Autodesk Inventor part; units mm, degrees
ref_plane "YZ Plane" through (0, 0, 0) normal (1, 0, 0) x (0, 1, 0)
ref_plane "XZ Plane" through (0, 0, 0) normal (0, 1, 0) x (-1, 0, 0)
ref_plane "XY Plane" through (0, 0, 0) normal (0, 0, 1) x (1, 0, 0)
sketch "Sketch1" plane through (0, 0, 0) normal (1, 0, 0) x (0, 1, 0)
  circle A0 centre (0, 0) radius 22.5
  circle A1 centre (0, 0) radius 8.375
  line L0 (8.375, 0) -> (22.5, 0) construction
  line L1 (22.1638, 3.875) -> (7.4246, 3.875) construction
  line L2 (7.4246, -3.875) -> (22.1638, -3.875) construction
  circle A2 centre (-14, 0) radius 3.0375
  circle A3 centre (-4.3262, -13.3148) radius 3.0375
  circle A4 centre (11.3262, -8.229) radius 3.0375
  circle A5 centre (11.3262, 8.229) radius 3.0375
  circle A6 centre (-4.3262, 13.3148) radius 3.0375
  dimension "d0" = 45
  dimension "d1" = 16.75
  dimension "d2" = 7.75
  dimension "d3" = 3.875
  dimension "d4" = 0
  dimension "d5" = 6.075
  dimension "d32" = 14
  dimension "d35" = 360
extrude "Extrusion1" add sketch "Sketch1" along normal blind 2
sketch "Sketch2" plane through (0, 0, 0) normal (-1, 0, 0) x (0, 0, 1)
  circle A0 centre (0, 0) radius 8.375
  circle A1 centre (0, 0) radius 22.5
extrude "Extrusion2" add sketch "Sketch2" along normal blind 0.25
sketch "Sketch3" plane through (2, 0, 0) normal (1, 0, 0) x (0, 0, -1)
  line L0 (-3.1, 26.8099) -> (3.1, 26.8099)
  line L1 (3.1, 26.8099) -> (3.1, 14.5)
  line L2 (3.1, 14.5) -> (-3.1, 14.5)
  line L3 (-3.1, 14.5) -> (-3.1, 26.8099)
  circle A0 centre (0, 0) radius 22.5 construction
  line L4 (-2.05, 26.8099) -> (2.05, 26.8099)
  line L5 (2.05, 26.8099) -> (2.05, 14.5)
  line L6 (2.05, 14.5) -> (-2.05, 14.5)
  line L7 (-2.05, 14.5) -> (-2.05, 26.8099)
  line L8 (-26.4557, 5.3365) -> (-24.5398, 11.233)
  line L9 (-24.5398, 11.233) -> (-12.8324, 7.429)
  line L10 (-12.8324, 7.429) -> (-14.7483, 1.5325)
  line L11 (-14.7483, 1.5325) -> (-26.4557, 5.3365)
  line L12 (-26.1313, 6.3351) -> (-24.8643, 10.2344)
  line L13 (-24.8643, 10.2344) -> (-13.1568, 6.4304)
  line L14 (-13.1568, 6.4304) -> (-14.4238, 2.5311)
  line L15 (-14.4238, 2.5311) -> (-26.1313, 6.3351)
  line L16 (-13.2505, -23.5118) -> (-18.2664, -19.8676)
  line L17 (-18.2664, -19.8676) -> (-11.0308, -9.9086)
  line L18 (-11.0308, -9.9086) -> (-6.0149, -13.5529)
  line L19 (-6.0149, -13.5529) -> (-13.2505, -23.5118)
  line L20 (-14.1, -22.8947) -> (-17.417, -20.4847)
  line L21 (-17.417, -20.4847) -> (-10.1814, -10.5258)
  line L22 (-10.1814, -10.5258) -> (-6.8644, -12.9357)
  line L23 (-6.8644, -12.9357) -> (-14.1, -22.8947)
  line L24 (18.2664, -19.8676) -> (13.2505, -23.5118)
  line L25 (13.2505, -23.5118) -> (6.0149, -13.5529)
  line L26 (6.0149, -13.5529) -> (11.0308, -9.9086)
  line L27 (11.0308, -9.9086) -> (18.2664, -19.8676)
  line L28 (17.417, -20.4847) -> (14.1, -22.8947)
  line L29 (14.1, -22.8947) -> (6.8644, -12.9357)
  line L30 (6.8644, -12.9357) -> (10.1814, -10.5258)
  line L31 (10.1814, -10.5258) -> (17.417, -20.4847)
  line L32 (24.5398, 11.233) -> (26.4557, 5.3365)
  line L33 (26.4557, 5.3365) -> (14.7483, 1.5325)
  line L34 (14.7483, 1.5325) -> (12.8324, 7.429)
  line L35 (12.8324, 7.429) -> (24.5398, 11.233)
  line L36 (24.8643, 10.2344) -> (26.1313, 6.3351)
  line L37 (26.1313, 6.3351) -> (14.4238, 2.5311)
  line L38 (14.4238, 2.5311) -> (13.1568, 6.4304)
  line L39 (13.1568, 6.4304) -> (24.8643, 10.2344)
  dimension "d15" = 6.2
  dimension "d16" = 3.1
  dimension "d17" = 8
  dimension "d22" = 0
  dimension "d23" = 0
  dimension "d24" = 1.05
  dimension "d25" = 1.05
  dimension "d28" = 360
extrude "Extrusion3" cut sketch "Sketch3" against normal up to surface (2.25 mm away)
equation "\"d3\" = 0.5 * d2"
equation "\"d25\" = d24"
properties part number "Magnetic Disk"
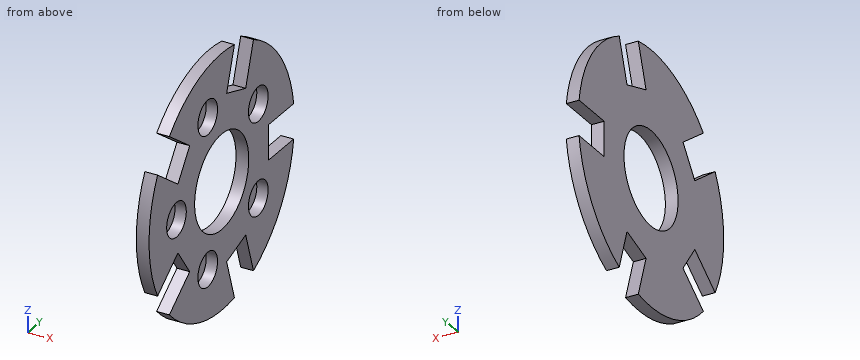
Build history of the part. All positions in model axes, mm. Round coordinates to 2 decimals unless told otherwise and drop trailing zeros. Order: outer loops, then holes, each group sorted by start corner. A loop starts at its lowest first (then second) coordinate and runs counter-clockwise, first axis right, second up. Notation, with made-up numbers: (89, 77.5) -> (111, 77.5) arc R13 cw to (111, 93.5) -> close; hole circle Ø11 at (-20.5, 79.5). An arc over 180 degrees is marked (long way). Answer in a Markdown table with one row per item.
1) Band-saw the part on A-A on y = -5.5. Give the cut face in (x, z), and give its area (3 significant figures).
Values:
| item | result |
|---|---|
| outline | (-0.25, -21.82) -> (2, -21.82) -> (2, -16.12) -> (0, -16.12) -> (0, -10.51) -> (2, -10.51) -> (2, -6.32) -> (-0.25, -6.32) -> close; (-0.25, 6.32) -> (2, 6.32) -> (2, 10.51) -> (0, 10.51) -> (0, 16.12) -> (2, 16.12) -> (2, 21.82) -> (-0.25, 21.82) -> close |
| area | 47.3 mm2 |
2) Wall check: L1, parallel to Z at x = 1.1, y = -16; L2, parallel to Y at x = 0.95, z = 10; L3, parallel to Y at x = 1.45, z = 5.5. Give the ranges that are in metal, low to high.
Values:
| item | result |
|---|---|
| L1 | -15.82 to -15.46, -7.79 to -2.29, 2.29 to 7.79, 15.46 to 15.82 |
| L2 | -20.16 to -19.04, -10.66 to 8.86, 13.79 to 20.16 |
| L3 | -21.82 to -6.32, 6.32 to 9.99, 12.66 to 21.82 |
3) Band-saw the part on B-B on x = 1.4. Give the number of separate pieces and of enclosed holes in the cut face, and give its area (3 significant figures).
Values:
| item | result |
|---|---|
| separate pieces | 1 |
| enclosed holes | 6 |
| area | 979 mm2 |
4) Band-saw the part on D-D on y = 15.5. Give the cut face in (x, z).
Values:
| item | result |
|---|---|
| outline | (-0.25, -16.31) -> (2, -16.31) -> (2, -3.1) -> (-0.25, -3.1) -> close; (-0.25, 3.1) -> (2, 3.1) -> (2, 16.31) -> (-0.25, 16.31) -> close |
5) Pin check, flat tips, straight feed: P1, Ø5, axis at y = -4.33, z = 13.31, coming from the +X side; P2, Ø0.7, axis at x = 1.5, z = -0.5, coming from the +Y side. Stop position of each tip, or through.
Values:
| item | result |
|---|---|
| P1 | x = 0 |
| P2 | y = 14.5 |
